Verification items for the finished model (mm, model axes). Round coordinates to 2 decimals unless told otherwise and drop trailing zeros. Loops run counter-clockwise (first coordinate to the right, second up) from the corner with the lowest first, then second, coordinate; pieces in that order, holes last. Notation, with made-up numbers: (70, 72) - (97, 72) arc R11 ccw to (97, 78) - close; hole circle Ø3 at (27, 19.5). An arc over 180 degrees is marked (long way). Use CSV: the item, a comma, the result in double quotes.
```python
from build123d import *

# Parameters (mm, degrees)
F0_W     = 101.6
F0_H     = 304.8
F1_DEPTH = 3.175
F3_D     = 6.35


# Not quite as in the source:
# - a length typed as a fraction of an inch, garbled in the dataset ("3 / 203.2 mm" for 3/8 in), is restored


with BuildPart() as f1:
    # F0 (on Top) → F1 (new body)
    with BuildSketch(Plane.XY):
        Rectangle(F0_W, F0_H)
    extrude(amount=F1_DEPTH)

    # F3 (through all)
    with Locations(Plane.XY.offset(3.175)):
        with Locations((-31.75, 133.35), (31.75, 133.35), (31.75, -120.65), (-31.75, -120.65), (0, 6.35), (-31.75, 110.49), (31.75, 110.49)):
            Hole(F3_D / 2)


solid = f1.part
```
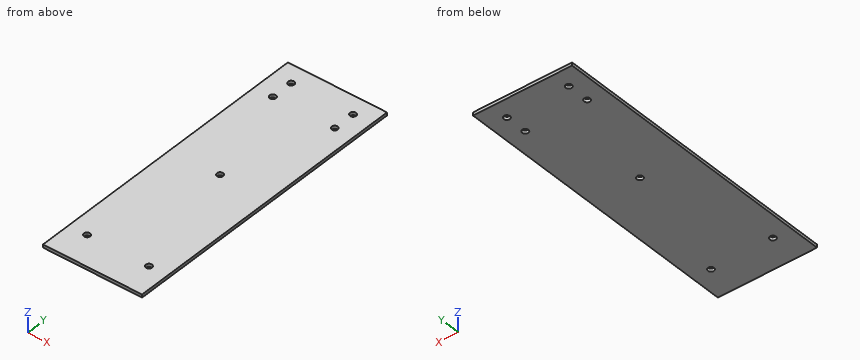
1) Thickness scan on probe 1 along Y at (x, z) = (31.75, 2) (3 decimals); probe 2 along X at (y, z) = (133.35, 0.7) (3 decimals); probe 3 along X at (y, z) = (-123, 1.6). Record the ranges inside material, lowest first. Write a range as [from, to].
Returned:
probe 1,"y = [-152.4, -123.825], [-117.475, 107.315], [113.665, 130.175], [136.525, 152.4]"
probe 2,"x = [-50.8, -34.925], [-28.575, 28.575], [34.925, 50.8]"
probe 3,"x = [-50.8, -33.88], [-29.62, 29.62], [33.88, 50.8]"
2) Cross-section at D-D, the plane y = 6.35. Record the cut outline in (x, z) (3 decimals), then the cut area to 3 significant figures.
Returned:
outline,"(-50.8, 0) - (-3.175, 0) - (-3.175, 3.175) - (-50.8, 3.175) - close; (3.175, 0) - (50.8, 0) - (50.8, 3.175) - (3.175, 3.175) - close"
area,"302 mm²"
3) Cross-section at B-B, the plane x = -31.75. Record the cut outline in (y, z) (3 decimals).
Returned:
outline,"(-152.4, 0) - (-123.825, 0) - (-123.825, 3.175) - (-152.4, 3.175) - close; (-117.475, 0) - (107.315, 0) - (107.315, 3.175) - (-117.475, 3.175) - close; (113.665, 0) - (130.175, 0) - (130.175, 3.175) - (113.665, 3.175) - close; (136.525, 0) - (152.4, 0) - (152.4, 3.175) - (136.525, 3.175) - close"
4) Cross-section at A-A, the plane x = 0. Record the cut outline in (y, z) (3 decimals).
Returned:
outline,"(-152.4, 0) - (3.175, 0) - (3.175, 3.175) - (-152.4, 3.175) - close; (9.525, 0) - (152.4, 0) - (152.4, 3.175) - (9.525, 3.175) - close"
5) Cross-section at C-C, the plane y = 133.35. Record the cut outline in (x, z) (3 decimals), then the cut area to 3 significant figures.
Returned:
outline,"(-50.8, 0) - (-34.925, 0) - (-34.925, 3.175) - (-50.8, 3.175) - close; (-28.575, 0) - (28.575, 0) - (28.575, 3.175) - (-28.575, 3.175) - close; (34.925, 0) - (50.8, 0) - (50.8, 3.175) - (34.925, 3.175) - close"
area,"282 mm²"
